Here's how the part is built. I have some questions about the finished solid (model axes, mm). Face numbers are marked on the shaded views. A direction names the side the tool comes from. Round coordinates to 2 decimals unless told otherwise and drop trailing zeros. Loops run counter-clockwise (first coordinate to the right, second up) from the corner with the lowest first, then second, coordinate; pieces in that order, holes last. Notation, with made-up numbers: M -33,12.5 L -7,12.5 A21 ccw -7,36.5 Z; hole C -33.5,-15 d5. An arc over 180 degrees is marked long. Answer as a JSON object with one key per item and string values.
from build123d import *

# Parameters (mm, degrees)
SKETCH022_R             = 18.5
PAD015_DEPTH            = 22
SKETCH023_R             = 17.5
PAD016_DEPTH            = 40
SKETCH024_R             = 6
PAD017_DEPTH            = 6
FILLET001_R             = 1
SKETCH025_R             = 3
PAD018_DEPTH            = 15
POCKET005_DEPTH         = 12
SKETCH027_R             = 1.5
POCKET006_DEPTH         = 15
BODY002_PLACEMENT_ANGLE = 90


with BuildPart() as part:
    # Sketch022 → Pad015 (new body)
    with BuildSketch(Plane.XZ):
        with Locations((0, 18.5)):
            Circle(SKETCH022_R)
    extrude(amount=PAD015_DEPTH)

    # Sketch023 (on Face3 of Pad015) → Pad016 (join)
    with BuildSketch(Plane.XZ.offset(22)):
        with Locations((0, 18.5)):
            Circle(SKETCH023_R)
    extrude(amount=PAD016_DEPTH)

    # Sketch024 (on Face2 of Pad016) → Pad017 (join)
    with BuildSketch(Plane(origin=(0, 0, 0), x_dir=(1, 0, 0), z_dir=(0, 1, 0))):
        with Locations((0, -25.5)):
            Circle(SKETCH024_R)
    extrude(amount=PAD017_DEPTH)

    # Fillet001
    fillet001_edges = [part.edges().sort_by_distance(p)[0] for p in [
        (-6, 6, 25.5),
    ]]
    fillet(fillet001_edges, radius=FILLET001_R)

    # Sketch025 (on Face4 of Fillet001) → Pad018 (join)
    with BuildSketch(Plane(origin=(0, 6, 0), x_dir=(1, 0, 0), z_dir=(0, 1, 0))):
        with Locations((0, -25.5)):
            Circle(SKETCH025_R)
    extrude(amount=PAD018_DEPTH)

    # Sketch026 (on Face8 of Pad018) → Pocket005 (cut)
    with BuildSketch(Plane(origin=(0, 21, 0), x_dir=(1, 0, 0), z_dir=(0, 1, 0))):
        with BuildLine():
            Line((-1.658312, -28), (1.658312, -28))
            ThreePointArc((-1.658312, -28), (0, -28.5), (1.658312, -28))
        make_face()
    extrude(amount=-POCKET005_DEPTH, mode=Mode.SUBTRACT)

    # Sketch027 (on Face3 of Pocket005) → Pocket006 (cut)
    with BuildSketch(Plane(origin=(0, 0, 0), x_dir=(1, 0, 0), z_dir=(0, 1, 0))):
        with Locations((-7.75, -5.08)):
            Circle(SKETCH027_R)
        with Locations((7.75, -5.08)):
            Circle(SKETCH027_R)
        with Locations((-15.5, -18.5)):
            Circle(SKETCH027_R)
        with Locations((15.5, -18.5)):
            Circle(SKETCH027_R)
        with Locations((7.75, -31.92)):
            Circle(SKETCH027_R)
        with Locations((-7.75, -31.92)):
            Circle(SKETCH027_R)
    extrude(amount=-POCKET006_DEPTH, mode=Mode.SUBTRACT)


with BuildPart() as part_1:
    # Body002 placement: moved
    add(part.part.moved(Location((454, -66.5, 0))).rotate(Axis((454, -66.5, 0), (0, 1, 0)), BODY002_PLACEMENT_ANGLE))


solid = part_1.part
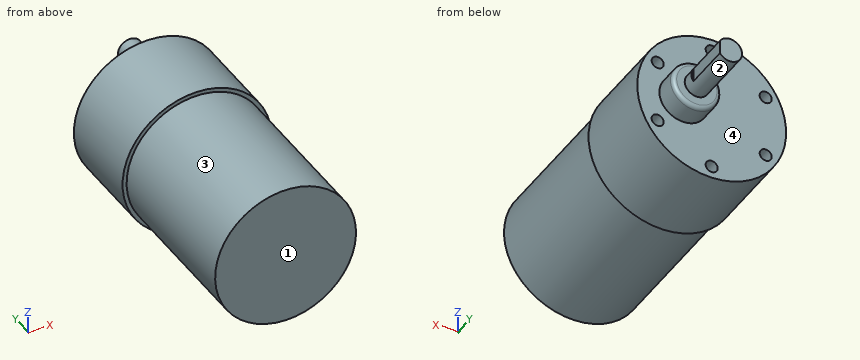
Item 1: If we mould it in two halves opening along Z, with no side actions, what happens to the marked faces 3 and 4? For each: pulls with the +Z half, pulls with the -Z half, needs draft (parallel to the pull), parting line crosses it, or undercut.
Resolved:
{"face 3": "parting line crosses it", "face 4": "needs draft"}
Item 2: I want a section at A-A, the plane y = -68. Please give me the cut outline in (x, z), then the cut area to 3 significant figures.
Resolved:
{"outline": "C 472.5,0 d37; hole C 459.08,-7.75 d3; hole C 459.08,7.75 d3; hole C 472.5,-15.5 d3; hole C 472.5,15.5 d3; hole C 485.92,-7.75 d3; hole C 485.92,7.75 d3", "area": "1,030 mm²"}
Item 3: On a 3-axis mill with a long thin cutter (end or side, diameter ignored), from which of +Z, -Z, +X, -X, +Y, -Y can I reach the whole of each face in a straight line? I mean the marked faces 1 and 2. Say none if no direction works.
Resolved:
{"face 1": "+Z, -Z, +X, -X, -Y", "face 2": "+Y"}
Item 4: I want a section at D-D, the plane y = -108.5. Please give me the cut outline in (x, z).
Resolved:
{"outline": "C 472.5,0 d35"}
Item 5: I'm going to push flat-ended pins straight in: pin 1 Ø4 at (x, z) = (459.08, -7.75) entering from +Y; pin 2 Ø2.5 at (x, z) = (485.92, 7.75) entering from +Y; pin 3 Ø1 at (y, z) = (-102, -5.5) entering from +X. Where does each tip first touch, or does it pass through?
Resolved:
{"pin 1": "y = -66.5", "pin 2": "y = -81.5", "pin 3": "x = 489.27"}
Item 6: Please list where these lines run through material, in increasing order: probe 1 along X at (y, z) = (-78.5, 7.75); probe 2 along Z at (x, y) = (472, -71); probe 3 along Z at (x, y) = (459.08, -71). Write a range as from..to.
Resolved:
{"probe 1": "455.7..457.58, 460.58..484.42, 487.42..489.3", "probe 2": "-18.49..-16.91, -14.09..14.09, 16.91..18.49", "probe 3": "-12.73..-9.25, -6.25..6.25, 9.25..12.73"}
Item 7: I want a section at B-B, the plane x = 472.5. Please give me the cut outline in (y, z), then the cut area to 3 significant figures.
Resolved:
{"outline": "M -128.5,-17.5 L -88.5,-17.5 L -88.5,-18.5 L -66.5,-18.5 L -66.5,-17 L -81.5,-17 L -81.5,-14 L -66.5,-14 L -66.5,14 L -81.5,14 L -81.5,17 L -66.5,17 L -66.5,18.5 L -88.5,18.5 L -88.5,17.5 L -128.5,17.5 Z", "area": "2,120 mm²"}
Item 8: I want a section at C-C, the plane z = 11. Please give me the cut outline in (x, y), then the cut area to 3 significant figures.
Resolved:
{"outline": "M 457.63,-88.5 L 458.89,-88.5 L 458.89,-128.5 L 486.11,-128.5 L 486.11,-88.5 L 487.37,-88.5 L 487.37,-66.5 L 457.63,-66.5 Z", "area": "1,740 mm²"}
